Could you check a few things on this model? Use its own coordinates, in mm. A direction names the side the tool comes from. Give positions to 0.01 mm unless a question says otherwise; leave off trailing zeros. Write each loop counter-clockwise with the first axis right and the second up, starting at its lowest first coordinate (ties: lowest second). Pieces come first, ordered by that corner, then holes. Notation, with made-up numbers: (-19, -9.75) - (-2, -9.75) arc R16 ccw to (-2, 5.25) - close; hole circle Ø8 at (89, 7.5). An arc over 180 degrees is marked (long way). Write item = value, one per line.
Autodesk Fusion 360 part; units mm, degrees
sketch "Sketch1" plane through (0, 0, 0) normal (0, 0, 1) x (1, 0, 0)
  line L0 (49, 49) -> (-49, 49) construction
  line L1 (-49, 49) -> (-49, -49) construction
  line L2 (-49, -49) -> (49, -49) construction
  line L3 (49, -49) -> (49, 49) construction
  line L4 (49, 49) -> (-49, -49) construction
  line L5 (-49, 49) -> (49, -49) construction
  line L6 (-34.6482, 34.6482) -> (-33.8425, 35.454)
  line L7 (-34.6482, 34.6482) -> (-20.2965, 49) construction
  line L8 (-34.6482, 34.6482) -> (-49, 20.2965) construction
  line L9 (-34.6482, -34.6482) -> (-49, -20.2965) construction
  line L10 (-34.6482, -34.6482) -> (-20.2965, -49) construction
  line L11 (34.6482, -34.6482) -> (20.2965, -49) construction
  line L12 (34.6482, -34.6482) -> (49, -20.2965) construction
  line L13 (34.6482, 34.6482) -> (49, 20.2965) construction
  line L14 (34.6482, 34.6482) -> (20.2965, 49) construction
  line L15 (-20.8111, 45.3788) -> (-11.5222, 47.626)
  line L16 (-28.9236, 45.6762) -> (-38.023, 48.5976)
  arc A0 (-28.9236, 45.6762) -> (-20.8111, 45.3788) centre (-24.3383, 59.9582) ccw
  arc A1 (-45.3788, 20.8111) -> (-45.6762, 28.9236) centre (-59.9582, 24.3383) ccw
  line L17 (-45.6762, 28.9236) -> (-48.5976, 38.023)
  line L18 (-45.3788, 20.8111) -> (-47.626, 11.5222)
  line L19 (-45.6762, -28.9236) -> (-48.5976, -38.023)
  line L20 (-28.9236, -45.6762) -> (-38.023, -48.5976)
  arc A2 (-20.8111, -45.3788) -> (-28.9236, -45.6762) centre (-24.3383, -59.9582) ccw
  line L21 (-20.8111, -45.3788) -> (-11.5222, -47.626)
  arc A3 (-45.6762, -28.9236) -> (-45.3788, -20.8111) centre (-59.9582, -24.3383) ccw
  line L22 (-45.3788, -20.8111) -> (-47.626, -11.5222)
  line L23 (28.9236, -45.6762) -> (38.023, -48.5976)
  line L24 (45.6762, -28.9236) -> (48.5976, -38.023)
  arc A4 (45.3788, -20.8111) -> (45.6762, -28.9236) centre (59.9582, -24.3383) ccw
  line L25 (45.3788, -20.8111) -> (47.626, -11.5222)
  arc A5 (28.9236, -45.6762) -> (20.8111, -45.3788) centre (24.3383, -59.9582) ccw
  line L26 (20.8111, -45.3788) -> (11.5222, -47.626)
  line L27 (45.6762, 28.9236) -> (48.5976, 38.023)
  line L28 (28.9236, 45.6762) -> (38.023, 48.5976)
  arc A6 (20.8111, 45.3788) -> (28.9236, 45.6762) centre (24.3383, 59.9582) ccw
  line L29 (20.8111, 45.3788) -> (11.5222, 47.626)
  arc A7 (45.6762, 28.9236) -> (45.3788, 20.8111) centre (59.9582, 24.3383) ccw
  line L30 (45.3788, 20.8111) -> (47.626, 11.5222)
  arc A8 (-38.023, 48.5976) -> (-48.5976, 38.023) centre (-40.5929, 40.5929) ccw
  arc A9 (-48.5976, -38.023) -> (-38.023, -48.5976) centre (-40.5929, -40.5929) ccw
  arc A10 (38.023, -48.5976) -> (48.5976, -38.023) centre (40.5929, -40.5929) ccw
  arc A11 (48.5976, 38.023) -> (38.023, 48.5976) centre (40.5929, 40.5929) ccw
  arc A12 (11.5222, 47.626) -> (-11.5222, 47.626) centre (0, 0) ccw
  arc A13 (47.626, -11.5222) -> (47.626, 11.5222) centre (0, 0) ccw
  arc A14 (-47.626, 11.5222) -> (-47.626, -11.5222) centre (0, 0) ccw
  arc A15 (-11.5222, -47.626) -> (11.5222, -47.626) centre (0, 0) ccw
  circle A16 centre (-40.5929, 40.5929) radius 2.5
  circle A17 centre (-40.5929, -40.5929) radius 2.5
  circle A18 centre (40.5929, -40.5929) radius 2.5
  circle A19 centre (40.5929, 40.5929) radius 2.5
  circle A20 centre (0, 0) radius 42.5 construction
  line L31 (0, 0) -> (16.6061, 39.1215) construction
  line L32 (0, 0) -> (42.5, 0) construction
  circle A21 centre (16.6061, 39.1215) radius 1.5
  circle A22 centre (-15.9208, 39.4053) radius 1.5
  circle A23 centre (-39.1215, 16.6061) radius 1.5
  circle A24 centre (-39.4053, -15.9208) radius 1.5
  circle A25 centre (-16.6061, -39.1215) radius 1.5
  circle A26 centre (15.9208, -39.4053) radius 1.5
  circle A27 centre (39.1215, -16.6061) radius 1.5
  circle A28 centre (39.4053, 15.9208) radius 1.5
  circle A29 centre (0, 0) radius 24.25
  dimension "d1" = 98
  dimension "d2" = 98
  dimension "d3" = 98
  dimension "d5" = 360
  dimension "d8" = 15
  dimension "d12" = 360
  dimension "d13" = 5
  dimension "d15" = 360
  dimension "d18" = 85
  dimension "d19" = 67
  dimension "d20" = 3
  dimension "d22" = 360
  dimension "d23" = 48.5
extrude "Extrude1" add sketch "Sketch1" along normal blind 3
chamfer "Chamfer1" distance 0.5 angle 45 1 faces at (24.2199, -1.2088, 2)
chamfer "Chamfer1" distance 0.25 angle 45 12 faces at (-38.096, 40.4683, 2) (-38.7152, 15.1621, 1) (-37.9072, -15.9955, 2) (-17.2381, 38.6879, 2) (17.886, 39.9036, 2) (39.8116, 14.4768, 1) (43.0898, 40.4683, 2) (43.0898, -40.7175, 2) (38.4371, -17.9409, 2) (17.2007, -38.6232, 2) (-17.9234, -39.8388, 2) (-38.096, -40.7175, 2)
equation "d3 = 120 mm - 2 mm - 20 mm"
equation "d19 = 90 deg - 23 deg"
1. If we section it at D-D, the plane x = -34: Please give me the cut outline in (y, z), and give its area (3 significant figures).
Filled sheet:
outline = (-47.31, 0) - (47.31, 0) - (47.31, 3) - (-47.31, 3) - close
area = 284 mm2
2. I need wall thicknesses on line 1 (X direction, y = 25, z = 0.6); line 2 (X direction, y = -19, z = 0.5); line 3 (Y direction, x = -2.5, z = 2.4). Which ranges of each line are inside material? Lowest first, please.
Filled sheet:
line_1 = -44.97 to 44.97
line_2 = -45.82 to -15.07, 15.07 to 45.82
line_3 = -48.94 to -24.12, 24.12 to 48.94
3. If we section it at C-C, the plane z = 1.6: Count the separate pieces of the cut face and the enclosed holes in it, and give its area (3 significant figures).
Filled sheet:
separate_pieces = 1
enclosed_holes = 13
area = 6,950 mm2
4. If we section it at A-A, the plane y = 0: Please give me the cut outline in (x, z), and give its area (3 significant figures).
Filled sheet:
outline = (-49, 0) - (-24.75, 0) - (-24.25, 0.5) - (-24.25, 2.5) - (-24.75, 3) - (-49, 3) - close; (24.25, 0.5) - (24.75, 0) - (49, 0) - (49, 3) - (24.75, 3) - (24.25, 2.5) - close
area = 148 mm2
5. Which directions (+Z, -Z, +X, -X, +Y, -Y) give clear straight access to the entire face, cutting with the end or side of a thin tool? Please do faces 1 (the face through (46.487, 16.232, 1.479)), 2 (the face through (42.98, -41.34, 1.48)), 3 (the face through (16.232, 46.487, 1.479)).
Filled sheet:
face_1 = +Z, -Z, +X
face_2 = +Z, -Z
face_3 = +Z, -Z, +Y
6. Thinking about a two-plate mould opening in X: for faces 4 (the face through (-37.975, -16.371, 1.482)), 5 (the face through (44.97, -24.95, 1.48)), 6 (the face through (-16.232, 46.487, 1.479)), which applies, pulls with the +X half, pulls with the -X half, needs draft (parallel to the pull), parting line crosses it, or undercut?
Filled sheet:
face_4 = undercut
face_5 = pulls with the +X half
face_6 = undercut
7. For pin 1 (2 mm diameter, centred on x = -2, y = 31, fed in from -Z); pin 2 (2.5 mm diameter, centred on x = 15.92, y = -39.41, fed in from +Z); pin 3 (1 mm diameter, centred on y = 38, z = 0.5, fed in from +X); pin 4 (3 mm diameter, centred on x = -22, y = 7, fed in from +Z), each with a flat end and sliding along its axis, tell me the tip position at first contact or that it passes through.
Filled sheet:
pin_1 = 0
pin_2 = through
pin_3 = 48.74
pin_4 = 2.84
